The listing builds one solid part. Answer for the finished solid, in the listing's coordinates (mm). Face numbers are marked on the shaded views. Coordinates: 2 decimals unless noted, no trailing zeros. Order: outer loops, then holes, each group sorted by start corner. A loop starts at its lowest first (then second) coordinate and runs counter-clockwise, first axis right, second up.
from build123d import *

# Parameters (mm, degrees)
FILLET1_R = 4


with BuildPart() as part:
    # Sketch1 → Revolve1 (revolve)
    with BuildSketch(Plane.XY, mode=Mode.PRIVATE) as revolve1_sk:
        with BuildLine():
            ThreePointArc((12.609380103, 0), (10.129852422, -0.034707115), (8.9, -2.188012744))
            Line((8.9, -2.188012744), (8.9, -27.380086709))
            Line((8.9, -27.380086709), (0, -27.380086709))
            Line((0, -27.380086709), (0, -75))
            Line((0, -75), (22, -75))
            Line((22, -75), (11.4, -22.688012744))
            Line((11.4, -22.688012744), (11.4, -4.688012744))
            ThreePointArc((11.4, -4.688012744), (13.820746978, -2.81249979), (12.609380103, 0))
        make_face()
    revolve(revolve1_sk.sketch.rotate(Axis((0, -27.380086709, 0), (0, -1, 0)), 180), axis=Axis((0, -27.380086709, 0), (0, -1, 0)))

    # Fillet1
    fillet1_edges = [part.edges().sort_by_distance(p)[0] for p in [
        (22, -75, 0),
    ]]
    fillet(fillet1_edges, radius=FILLET1_R)


solid = part.part
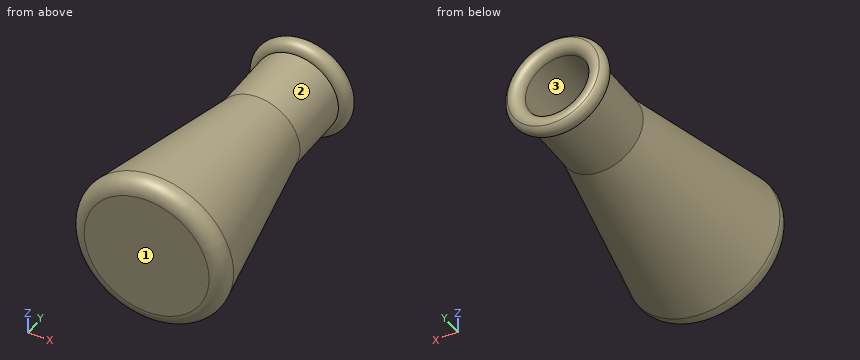
1) Section A-A (y = -10.5) is taken. Give the vertices of the cut face in (x, z), then the cut area to 3 significant figures.
2) Consider L1, parallel to Z at x = 0, y = -20.75; L2, parallel to X at y = -23, z = -7.5; L3, parallel to Y at x = 8, z = 3. Determine where each line is inside the solid, lowest interval first.
3) Determine the mould class of the marked faces 1, 2 and 3 for opening direction Y: released by +Y, released by -Y, zero draft, split by the parting line, or undercut.
4) Each of these flat-tipped pins is pushed along its axis until it touches: P1, Ø6, axis at y = -56.5, z = -7, coming from the -X side; P2, Ø8, axis at x = 0.5, y = -67, coming from the -Z side; P3, Ø14, axis at x = -3.5, z = -1.5, coming from the +Y side. Where does it stop, or does it pass through?
5) Section B-B (y = -45.5) is taken. Give the vertices of the cut face in (x, z).
Filled sheet:
1. outline: circle Ø22.8 at (0, 0); hole circle Ø17.8 at (0, 0)
1. area: 159 mm2
2. L1: z = -11.4 to -8.9, 8.9 to 11.4
2. L2: x = -8.67 to -4.79, 4.79 to 8.67
2. L3: y = -75 to -27.38
3. face 1: released by -Y
3. face 2: undercut
3. face 3: zero draft
4. P1: stops at x = -18.04
4. P2: stops at z = -21.11
4. P3: stops at y = 0.24
5. outline: circle Ø32.04 at (0, 0)
